Work out the finished part from the listing and answer in its coordinate system (mm). A direction names the side the tool comes from. Give positions to 0.01 mm unless a question says otherwise; leave off trailing zeros. Loops run counter-clockwise (first coordinate to the right, second up) from the corner with the lowest first, then second, coordinate; pieces in that order, holes last. Notation, with made-up numbers: (-14.75, -7) - (44.25, -7) arc R15 ccw to (44.25, 2) - close; hole circle Ø10 at (-22.5, 69). An arc over 180 degrees is marked (long way). One line per question, with ' | ' between items. Start each with the question number.
1. Each of these flat-tipped pins is pushed along its axis until it touches: pin 1 (8 mm diameter, centred on x = -1, y = -5, fed in from -Z); pin 2 (1.5 mm diameter, centred on y = 11.5, z = 2.5, fed in from +X); pin 3 (5 mm diameter, centred on y = -9.5, z = 11, fed in from +X); pin 4 (10 mm diameter, centred on x = -14.5, y = -12, fed in from +Z). Where does it stop, or does it pass through?
2. Section B-B (y = 9) is taken. Determine the outline of the cut face in (x, z).
3. Section A-A (x = 0) is taken. Determine the outline of the cut face in (y, z), plus the area to 3 significant figures.
4. For a pull along Y with two mould halves and no side action, classify faces 1 (the face through (-11.88, -17.84, 8.7)), 2 (the face through (-5, 19, 10)), 3 (the face through (0, -19.284, 3)) as released by +Y, released by -Y, zero draft, split by the parting line, or undercut.
5. Section D-D (y = -23.5) is taken. Determine the outline of the cut face in (x, z).
6. Find the intervals of material crossed by line 1 (X direction, y = 15.25, z = 1.05); line 2 (Z direction, x = 9, y = -16.5), in increasing order.
7. Which of the six approach directions +Z, -Z, +X, -X, +Y, -Y give full straight-line access (tool end or side, diameter ignored) to faces 4 (the face through (11.87, -17.88, 8.7)), 5 (the face through (0, 19, 1)), 6 (the face through (0, 0, 1.5))?
8. Section C-C (x = 8.5) is taken. Determine the outline of the cut face in (y, z).
from build123d import *

# Parameters (mm, degrees)
PRINT_2_DEPTH        = 1.5
PRINT_HOLES_REACH    = 28.912
SKETCH1_4_R          = 1.25
SKETCH1_5_R          = 1.75
SCREWS_DEPTH         = 3
SKETCH1_6_W          = 21
SKETCH1_6_H          = 5.5
CABLECONNECTOR_DEPTH = 3
CAM_START            = 1.5
CAM_BASE_DEPTH       = 11
BASE_START           = 12.5
SKETCH1_8_W          = 10
SKETCH1_8_H          = 4
BASE_CLAMP_DEPTH     = 5
BOSS_EXTRUDE6_START  = 5
BOSS_EXTRUDE6_DEPTH  = 7.5
BOSS_EXTRUDE7_START  = 12.5
SKETCH1_10_W         = 14
SKETCH1_10_H         = 8
SKETCH1_10_H_2       = 3
BOSS_EXTRUDE7_DEPTH  = 11.5


with BuildPart() as part:
    # Sketch1 → print 2 (new body)
    with BuildSketch(Plane.XY):
        with BuildLine():
            Line((-15, -19), (15, -19))
            ThreePointArc((15, -19), (17.828427125, -17.828427125), (19, -15))
            Line((19, -15), (19, 15))
            ThreePointArc((19, 15), (17.828427125, 17.828427125), (15, 19))
            Line((15, 19), (-15, 19))
            ThreePointArc((-15, 19), (-17.828427125, 17.828427125), (-19, 15))
            Line((-19, 15), (-19, -15))
            ThreePointArc((-19, -15), (-17.828427125, -17.828427125), (-15, -19))
        make_face()
    extrude(amount=PRINT_2_DEPTH)

    # Sketch1<4> → print_holes (cut, up to next)
    with BuildSketch(Plane.XY, mode=Mode.PRIVATE) as print_holes_sk1:
        with Locations((-15.25, 15.25)):
            Circle(SKETCH1_4_R)
    print_holes_tool1 = extrude(print_holes_sk1.sketch, amount=PRINT_HOLES_REACH, mode=Mode.PRIVATE) & part.part
    # Sketch1<4> → print_holes (cut, up to next)
    with BuildSketch(Plane.XY, mode=Mode.PRIVATE) as print_holes_sk2:
        with Locations((-15.25, -15.25)):
            Circle(SKETCH1_4_R)
    print_holes_tool2 = extrude(print_holes_sk2.sketch, amount=PRINT_HOLES_REACH, mode=Mode.PRIVATE) & part.part
    # Sketch1<4> → print_holes (cut, up to next)
    with BuildSketch(Plane.XY, mode=Mode.PRIVATE) as print_holes_sk3:
        with Locations((15.25, -15.25)):
            Circle(SKETCH1_4_R)
    print_holes_tool3 = extrude(print_holes_sk3.sketch, amount=PRINT_HOLES_REACH, mode=Mode.PRIVATE) & part.part
    # Sketch1<4> → print_holes (cut, up to next)
    with BuildSketch(Plane.XY, mode=Mode.PRIVATE) as print_holes_sk4:
        with Locations((15.25, 15.25)):
            Circle(SKETCH1_4_R)
    print_holes_tool4 = extrude(print_holes_sk4.sketch, amount=PRINT_HOLES_REACH, mode=Mode.PRIVATE) & part.part
    add(print_holes_tool1.solids().sort_by_distance((-15.25, 15.25, 0))[0], mode=Mode.SUBTRACT)
    add(print_holes_tool2.solids().sort_by_distance((-15.25, -15.25, 0))[0], mode=Mode.SUBTRACT)
    add(print_holes_tool3.solids().sort_by_distance((15.25, -15.25, 0))[0], mode=Mode.SUBTRACT)
    add(print_holes_tool4.solids().sort_by_distance((15.25, 15.25, 0))[0], mode=Mode.SUBTRACT)

    # Sketch1<5> → screws (add)
    with BuildSketch(Plane.XY):
        with Locations((-12.25, 0)):
            Circle(SKETCH1_5_R)
        with Locations((12.25, 0)):
            Circle(SKETCH1_5_R)
    extrude(amount=-SCREWS_DEPTH)

    # Sketch1<6> → cableconnector (add)
    with BuildSketch(Plane.XY):
        with Locations((0, -16.25)):
            Rectangle(SKETCH1_6_W, SKETCH1_6_H)
    extrude(amount=-CABLECONNECTOR_DEPTH)

    # Sketch1<7> → cam base (add)
    with BuildSketch(Plane.XY.offset(CAM_START)):
        with BuildLine():
            ThreePointArc((-5, 16.770509831), (-17.226972131, 3.079193268), (-10.5, -14))
            Line((-10.5, -14), (-10.5, -13.5))
            Line((-10.5, -13.5), (-3.708099244, -13.5))
            ThreePointArc((-3.708099244, -13.5), (-11.133584092, -8.487832778), (-14, 5e-09))
            ThreePointArc((-14, 5e-09), (2e-09, 14), (14, 0))
            ThreePointArc((14, 0), (11.133584091, -8.48783278), (3.708099244, -13.5))
            Line((3.708099244, -13.5), (10.5, -13.5))
            Line((10.5, -13.5), (10.5, -14))
            ThreePointArc((10.5, -14), (15.652475842, -7.826237921), (17.5, 0))
            ThreePointArc((17.5, 0), (14.0312152, 10.458250332), (5, 16.770509831))
            Line((5, 16.770509831), (-5, 16.770509831))
        make_face()
        with BuildLine():
            Line((-10.5, -13.5), (-10.5, -14))
            ThreePointArc((-10.5, -14), (-10.251592739, -14.182906836), (-10, -14.361406616))
            ThreePointArc((-10, -14.361406616), (0, -17.5), (10, -14.361406616))
            ThreePointArc((10, -14.361406616), (10.251592739, -14.182906836), (10.5, -14))
            Line((10.5, -14), (10.5, -13.5))
            Line((10.5, -13.5), (3.708099244, -13.5))
            ThreePointArc((3.708099244, -13.5), (0, -14), (-3.708099244, -13.5))
            Line((-3.708099244, -13.5), (-10.5, -13.5))
        make_face()
        with BuildLine():
            ThreePointArc((5, 16.770509831), (0, 17.5), (-5, 16.770509831))
            Line((-5, 16.770509831), (5, 16.770509831))
        make_face()
    extrude(amount=CAM_BASE_DEPTH)

    # Sketch1<8> → base clamp (add)
    with BuildSketch(Plane.XY.offset(BASE_START)):
        with Locations((0, 18.770509831)):
            Rectangle(SKETCH1_8_W, SKETCH1_8_H)
    extrude(amount=-BASE_CLAMP_DEPTH)

    # Sketch1<9> → Boss-Extrude6 (add)
    with BuildSketch(Plane.XY.offset(BOSS_EXTRUDE6_START)):
        with BuildLine():
            Line((-11.5, -19.361406616), (-7, -22.283740786))
            Line((-7, -22.283740786), (-7, -19.283740786))
            Line((-7, -19.283740786), (7, -19.283740786))
            Line((7, -19.283740786), (7, -22.283740786))
            Line((7, -22.283740786), (11.5, -19.361406616))
            Line((11.5, -19.361406616), (12.25, -16.361406616))
            Line((12.25, -16.361406616), (10, -14.361406616))
            ThreePointArc((10, -14.361406616), (0, -17.5), (-10, -14.361406616))
            Line((-10, -14.361406616), (-12.25, -16.361406616))
            Line((-12.25, -16.361406616), (-11.5, -19.361406616))
        make_face()
    extrude(amount=BOSS_EXTRUDE6_DEPTH)

    # Sketch1<10> → Boss-Extrude7 (add)
    with BuildSketch(Plane.XY.offset(BOSS_EXTRUDE7_START)):
        with Locations((0, -26.283740786)):
            Rectangle(SKETCH1_10_W, SKETCH1_10_H)
        with Locations((0, -20.783740786)):
            Rectangle(SKETCH1_10_W, SKETCH1_10_H_2)
    extrude(amount=-BOSS_EXTRUDE7_DEPTH)


solid = part.part
Conclusion:
1) pin 1: z = 0 | pin 2: x = 13.81 | pin 3: x = 16.04 | pin 4: z = 12.5
2) outline: (-19, 0) - (19, 0) - (19, 1.5) - (15.01, 1.5) - (15.01, 12.5) - (10.72, 12.5) - (10.72, 1.5) - (-10.72, 1.5) - (-10.72, 12.5) - (-15.01, 12.5) - (-15.01, 1.5) - (-19, 1.5) - close
3) outline: (-30.28, 1) - (-19.28, 1) - (-19.28, 5) - (-17.5, 5) - (-17.5, 1.5) - (-19, 1.5) - (-19, -3) - (-13.5, -3) - (-13.5, 0) - (19, 0) - (19, 1.5) - (17.5, 1.5) - (17.5, 7.5) - (20.77, 7.5) - (20.77, 12.5) - (14, 12.5) - (14, 1.5) - (-14, 1.5) - (-14, 12.5) - (-30.28, 12.5) - close | area: 307 mm²
4) face 1: released by -Y | face 2: zero draft | face 3: undercut
5) outline: (-7, 1) - (7, 1) - (7, 12.5) - (-7, 12.5) - close
6) line 1: -18.99 to -16.5, -14 to 14, 16.5 to 18.99 | line 2: -3 to 1.5, 5 to 12.5
7) face 4: +Z, +X, -Y | face 5: -Z, +X, -X, +Y | face 6: +Z
8) outline: (-21.31, 5) - (-15.3, 5) - (-15.3, 1.5) - (-19, 1.5) - (-19, -3) - (-13.5, -3) - (-13.5, 0) - (19, 0) - (19, 1.5) - (15.3, 1.5) - (15.3, 12.5) - (11.12, 12.5) - (11.12, 1.5) - (-11.12, 1.5) - (-11.12, 12.5) - (-21.31, 12.5) - close
